Input: dimensioned drawing with shaded views. Units: mm. Origin: part minimum x, y, z. A direction names the side the tool comes from. Give positions to 0.01 mm unless a question says otherwise; leave off trailing zeros. Write each loop counter-clockwise with the first axis right and the second up, starting at its lowest first coordinate (ties: lowest second). Pieces come first, ordered by that corner, then holes. Notation, with made-up numbers: (57.25, 33) -> (104.25, 33) arc R14 ccw to (104.25, 41) -> close; hole circle Ø4 at (-22, -5.5). An arc over 180 degrees is marked (long way). Answer as a JSON object with one key per item and string values. Group by question number.
(1) Draft query along Z for the marked faces 1, 2 and 3. Return one class per face: +Z half, -Z half, draft (parallel to the pull), parting line (faces both ways), or undercut.
(2) Section query B-B on z = 1.5. Output: boundary loops of the cut face in (x, y).
(3) Set-up query: the marked faces 4, 5 and 6. Return all of +Z, -Z, +X, -X, +Y, -Y with unobstructed straight access to the full face (end or side cutting, diameter ignored); none if empty.
(4) Contact query for flat-ended pins moving along their axis: pin 1 Ø3 at (x, z) = (35.5, 4) entering from +Y; pin 2 Ø2 at (y, z) = (8.5, 2) entering from -X; pin 3 Ø3 at (y, z) = (29.5, 4.5) entering from +X. Output: stop coordinate, or through.
(5) Material intervals for probe 1 along X at (y, z) = (5, 3.25); probe 2 along X at (y, z) = (16, 5); probe 3 along Y at (x, z) = (35.5, 6), sorted ascending.
(6) Section query C-C on y = 45. Output: boundary loops of the cut face in (x, z).
(7) Section query A-A on x = 19.05. Output: boundary loops of the cut face in (y, z), plus the area to 3 significant figures.
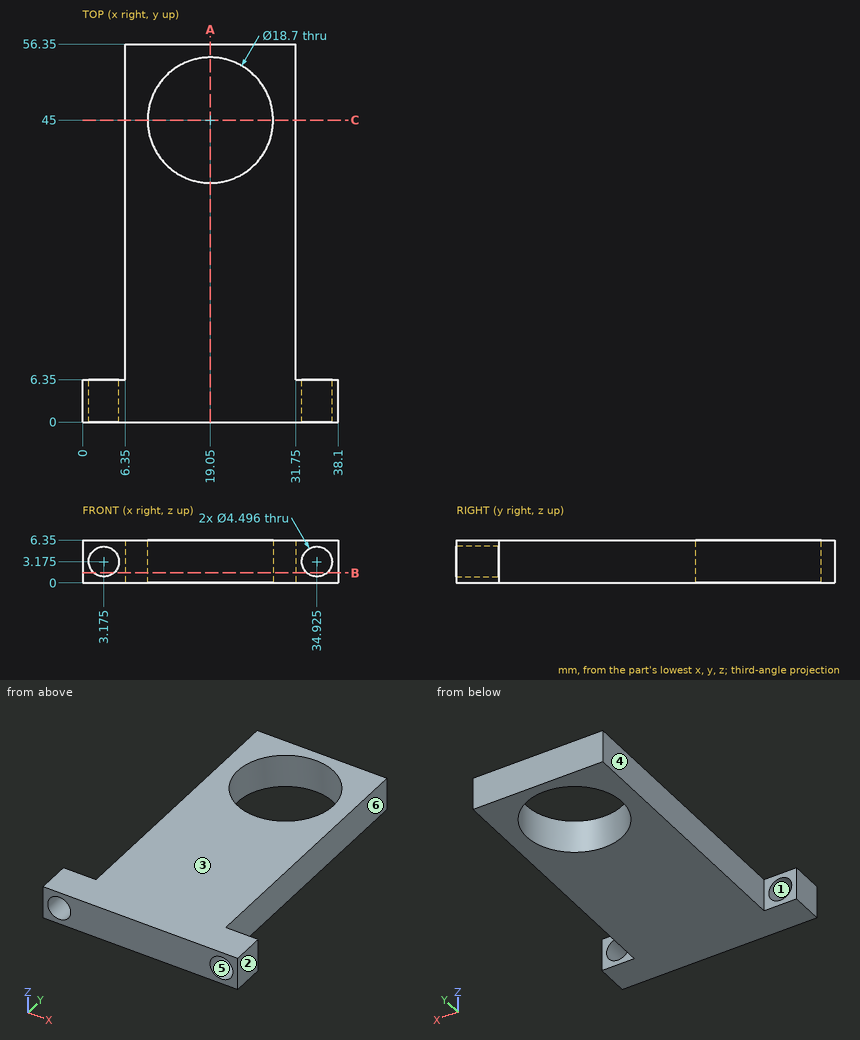
Answer list:
{
 "1": {"face 1": "undercut", "face 2": "draft", "face 3": "+Z half"},
 "2": {"outline": "(0, 0) -> (1.68, 0) -> (1.68, 6.35) -> (0, 6.35) -> close; (4.67, 0) -> (33.43, 0) -> (33.43, 6.35) -> (31.75, 6.35) -> (31.75, 56.35) -> (6.35, 56.35) -> (6.35, 6.35) -> (4.67, 6.35) -> close; (36.42, 0) -> (38.1, 0) -> (38.1, 6.35) -> (36.42, 6.35) -> close; hole circle Ø18.7 at (19.05, 45)"},
 "3": {"face 4": "+Z, -Z, -X, +Y", "face 5": "+Y, -Y", "face 6": "+Z, -Z, +X, +Y"},
 "4": {"pin 1": "y = 6.35", "pin 2": "x = 6.35", "pin 3": "x = 31.75"},
 "5": {"probe 1": "0 to 0.93, 5.42 to 32.68, 37.17 to 38.1", "probe 2": "6.35 to 31.75", "probe 3": "0 to 6.35"},
 "6": {"outline": "(6.35, 0) -> (9.7, 0) -> (9.7, 6.35) -> (6.35, 6.35) -> close; (28.4, 0) -> (31.75, 0) -> (31.75, 6.35) -> (28.4, 6.35) -> close"},
 "7": {"outline": "(0, 0) -> (35.65, 0) -> (35.65, 6.35) -> (0, 6.35) -> close; (54.35, 0) -> (56.35, 0) -> (56.35, 6.35) -> (54.35, 6.35) -> close", "area": "239 mm2"}
}
